Autodesk Inventor part; units mm, degrees
ref_plane "YZ Plane" through (0, 0, 0) normal (1, 0, 0) x (0, 1, 0)
ref_plane "XZ Plane" through (0, 0, 0) normal (0, 1, 0) x (-1, 0, 0)
ref_plane "XY Plane" through (0, 0, 0) normal (0, 0, 1) x (1, 0, 0)
sketch "Sketch1" plane through (0, 0, 0) normal (0, 1, 0) x (-1, 0, 0)
  circle A0 centre (0, 0) radius 28.5
  circle A1 centre (0, 0) radius 9
  circle A2 centre (11.875, 20.5681) radius 1.5875
  circle A3 centre (-11.875, 20.5681) radius 1.5875
  circle A4 centre (23.75, 0) radius 1.5875
  circle A5 centre (11.875, -20.5681) radius 1.5875
  circle A6 centre (-11.875, -20.5681) radius 1.5875
  circle A7 centre (-23.75, 0) radius 1.5875
  dimension "d5" = 3.175
  dimension "d6" = 20.5681
  dimension "d7" = 3.175
  dimension "d8" = 3.175
  dimension "d9" = 3.175
  dimension "d10" = 3.175
  dimension "d11" = 3.175
extrude "Extrusion1" add sketch "Sketch1" along normal blind 46
sketch "Sketch2" plane through (0, 46, 0) normal (0, 1, 0) x (1, 0, 0)
  line L0 (7.5157, 0) -> (3.7578, -6.5088)
  line L1 (3.7578, -6.5088) -> (-3.7578, -6.5088)
  line L2 (-3.7578, -6.5088) -> (-7.5157, 0)
  line L3 (-7.5157, 0) -> (-3.7578, 6.5088)
  line L4 (-3.7578, 6.5088) -> (3.7578, 6.5088)
  line L5 (3.7578, 6.5088) -> (7.5157, 0)
  circle A0 centre (0, 0) radius 28.5
  circle A1 centre (-11.875, -20.5681) radius 1.5875
  circle A2 centre (11.875, -20.5681) radius 1.5875
  circle A3 centre (-23.75, 0) radius 1.5875
  circle A4 centre (-11.875, 20.5681) radius 1.5875
  circle A5 centre (23.75, 0) radius 1.5875
  circle A6 centre (11.875, 20.5681) radius 1.5875
  dimension "d4" = 13.0175
extrude "Extrusion2" add sketch "Sketch2" against normal blind 46
sketch "Sketch3" plane through (0, 46, 0) normal (0, 1, 0) x (1, 0, 0)
  circle A0 centre (-11.875, 20.5681) radius 1.5875
  circle A1 centre (-11.875, 20.5681) radius 2.3812
  circle A2 centre (11.875, 20.5681) radius 1.5875
  circle A3 centre (11.875, 20.5681) radius 2.3812
  circle A4 centre (23.75, 0) radius 1.5875
  circle A5 centre (23.75, 0) radius 2.3813
  circle A6 centre (11.875, -20.5681) radius 1.5875
  circle A7 centre (11.875, -20.5681) radius 2.3813
  circle A8 centre (-11.875, -20.5681) radius 1.5875
  circle A9 centre (-11.875, -20.5681) radius 2.3812
  circle A10 centre (-23.75, 0) radius 1.5875
  circle A11 centre (-23.75, 0) radius 2.3812
  point P0 (0, 0)
  dimension "d12" = 4.7625
  dimension "d13" = 4.7625
  dimension "d14" = 4.7625
  dimension "d15" = 4.7625
  dimension "d16" = 4.7625
  dimension "d17" = 4.7625
extrude "Extrusion3" add sketch "Sketch3" along normal blind 2.3813 and the other way blind 48.3807 contours A0 | A1 | A2 | A3 | A4 | A5 | A6 | A7 | A8 | A9 | A10 | A11
sketch "Sketch4" plane through (11.875, -2.3806, 20.5681) normal (0, -1, 0) x (1, 0, 0)
  circle A0 centre (-11.875, -20.5681) radius 42.5802
extrude "Extrusion4" cut sketch "Sketch4" against normal blind 44.45
sketch "Sketch5" plane through (0, 42.0694, 0) normal (0, -1, 0) x (1, 0, 0)
  circle A0 centre (0, 0) radius 9.525
  circle A1 centre (0, 0) radius 31.269
  dimension "d24" = 19.05
extrude "Extrusion5" cut sketch "Sketch5" against normal blind 25.4
equation "\"d7\" = d5"
equation "\"d8\" = d5"
equation "\"d9\" = d5"
equation "\"d10\" = d5"
equation "\"d11\" = d5"
properties part number "new mech inside test"
For this review, take the finished solid that the model builds, in its own axes (mm). A direction names the side the tool comes from. Round coordinates to 2 decimals unless told otherwise and drop trailing zeros. Loops run counter-clockwise (first coordinate to the right, second up) from the corner with the lowest first, then second, coordinate; pieces in that order, holes last.
(1) We need section D-D (z = 7.5). Give the boundary of the cut face in (x, y).
Returned:
outline: (-5.87, 42.07) - (5.87, 42.07) - (5.87, 46) - (-5.87, 46) - close
(2) We need section B-B (y = 45). Give the boundary of the cut face in (x, z) (3 decimals).
Returned:
outline: circle Ø19.05 at (0, 0); hole (-7.516, 0) - (-3.758, -6.509) - (3.758, -6.509) - (7.516, 0) - (3.758, 6.509) - (-3.758, 6.509) - close
(3) We need section C-C (z = 5.5). Give the boundary of the cut face in (x, y), plus the area to 3 significant figures.
Returned:
outline: (-7.78, 42.07) - (-4.34, 42.07) - (-4.34, 46) - (-7.78, 46) - close; (4.34, 42.07) - (7.78, 42.07) - (7.78, 46) - (4.34, 46) - close
area: 27.0 mm2
(4) Tool access review of faces 1 (the flat face through (5.663, 44.062, 3.209)), 2 (the flat face through (4.1, 42.069, -6.22)): name each direction out of +Z, -Z, +X, -X, +Y, -Y from which nothing blocks a thin tool from reaching the whole face with its end or side.
Returned:
face 1: +Y, -Y
face 2: +Z, -Z, +X, -X, -Y
(5) Mouldability with a two-part tool opening along Z and no side actions: class faces 3 (the flat face through (-5.663, 44.062, -3.209)), 4 (the flat face through (-4.1, 46, -6.22)), 5 (the cylindrical face through (-7.559, 44.007, -5.796)) as released by +Z, released by -Z, zero draft, split by the parting line, or undercut.
Returned:
face 3: undercut
face 4: zero draft
face 5: split by the parting line
(6) We need section A-A (x = 0). Give the boundary of the cut face in (y, z) (3 decimals), plus the area to 3 significant figures.
Returned:
outline: (42.069, -9.525) - (46, -9.525) - (46, -6.509) - (42.069, -6.509) - close; (42.069, 6.509) - (46, 6.509) - (46, 9.525) - (42.069, 9.525) - close
area: 23.7 mm2
(7) Wall thickness on line 1 along Z through (x, y) = (7.25, 42.95); line 2 along Z through (x, y) = (-1.25, 45.6); line 3 along X through (y, z) = (45.65, 1): over which ranges is each line inside the solid? List them lowest first.
Returned:
line 1: z = -6.18 to -0.46, 0.46 to 6.18
line 2: z = -9.44 to -6.51, 6.51 to 9.44
line 3: x = -9.47 to -6.94, 6.94 to 9.47
(8) Clearance check with a flat-ended pin moving along its axis: P1, Ø3, axis at x = 5, z = 0.5, coming from the +Y side. State where the tip first meets the part, or that it passes through.
Returned:
P1: passes through
